Source: CAD feature listing. Evaluate the final solid. Frame: model axes, mm. Face numbers are marked on the shaded views. Coordinates: 2 decimals unless noted, no trailing zeros. Write each loop counter-clockwise with the first axis right and the second up, starting at its lowest first coordinate (ties: lowest second). Pieces come first, ordered by that corner, then holes. Notation, with made-up numbers: (40, 73) - (73, 73) arc R27 cw to (73, 100) - close; hole circle Ø7 at (-17.75, -0.5). An arc over 180 degrees is marked (long way). One line per item, written item: value.
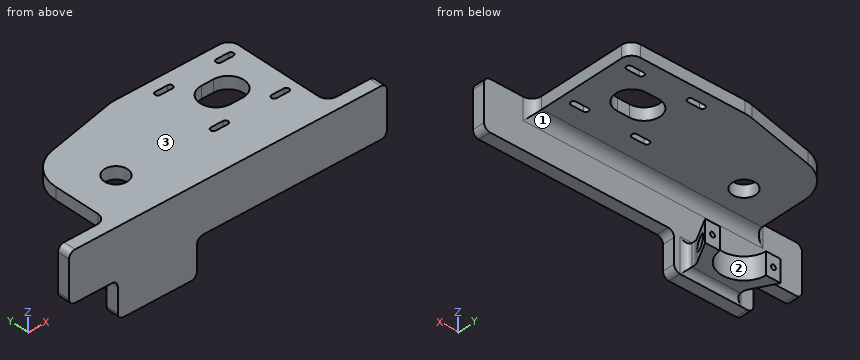
from build123d import *

# Parameters (mm, degrees)
SKETCH1_R           = 9.525
BOSS_EXTRUDE1_DEPTH = 10
SKETCH2_W           = 181
SKETCH2_H           = 100
BOSS_EXTRUDE2_DEPTH = 10
BOSS_EXTRUDE3_DEPTH = 18
SKETCH4_R           = 2
CUT_EXTRUDE1_DEPTH  = 30
SKETCH5_R           = 4
CUT_EXTRUDE2_DEPTH  = 20
CUT_EXTRUDE4_START  = -18
SKETCH8_W           = 62
SKETCH8_H           = 1
CUT_EXTRUDE4_DEPTH  = 18
CUT_EXTRUDE3_REACH  = 171.994
FILLET1_R           = 5
SKETCH9_W           = 40
SKETCH9_H           = 40
BOSS_EXTRUDE5_DEPTH = 10
CUT_EXTRUDE6_DEPTH  = 225.56428954
FILLET2_R           = 5
FILLET3_R           = 5
FILLET4_R           = 8
FILLET5_R           = 30


with BuildPart() as part:
    # Sketch1 → Boss-Extrude1 (new body)
    with BuildSketch(Plane.XY):
        Polygon((146, 57.938160866), (146, -30), (-35, -30), (-35, 40), (49, 57.938160866), align=None)
        Circle(SKETCH1_R, mode=Mode.SUBTRACT)
        with BuildLine():
            Line((101, 33.688160866), (111, 33.688160866))
            ThreePointArc((111, 33.688160866), (124, 20.688160866), (111, 7.688160866))
            Line((111, 7.688160866), (101, 7.688160866))
            ThreePointArc((101, 7.688160866), (88, 20.688160866), (101, 33.688160866))
        make_face(mode=Mode.SUBTRACT)
        with BuildLine():
            Line((86, 43.438160866), (76, 43.438160866))
            ThreePointArc((76, 43.438160866), (73.75, 45.688160866), (76, 47.938160866))
            Line((76, 47.938160866), (86, 47.938160866))
            ThreePointArc((86, 47.938160866), (88.25, 45.688160866), (86, 43.438160866))
        make_face(mode=Mode.SUBTRACT)
        with BuildLine():
            Line((86, -6.561839134), (76, -6.561839134))
            ThreePointArc((76, -6.561839134), (73.75, -4.311839134), (76, -2.061839134))
            Line((76, -2.061839134), (86, -2.061839134))
            ThreePointArc((86, -2.061839134), (88.25, -4.311839134), (86, -6.561839134))
        make_face(mode=Mode.SUBTRACT)
        with BuildLine():
            Line((126, -2.061839134), (136, -2.061839134))
            ThreePointArc((136, -2.061839134), (138.25, -4.311839134), (136, -6.561839134))
            Line((136, -6.561839134), (126, -6.561839134))
            ThreePointArc((126, -6.561839134), (123.75, -4.311839134), (126, -2.061839134))
        make_face(mode=Mode.SUBTRACT)
        with BuildLine():
            Line((126, 47.938160866), (136, 47.938160866))
            ThreePointArc((136, 47.938160866), (138.25, 45.688160866), (136, 43.438160866))
            Line((136, 43.438160866), (126, 43.438160866))
            ThreePointArc((126, 43.438160866), (123.75, 45.688160866), (126, 47.938160866))
        make_face(mode=Mode.SUBTRACT)
    extrude(amount=BOSS_EXTRUDE1_DEPTH)

    # Sketch2 → Boss-Extrude2 (add)
    with BuildSketch(Plane.XZ.offset(30)):
        with Locations((55.5, -40)):
            Rectangle(SKETCH2_W, SKETCH2_H)
    extrude(amount=BOSS_EXTRUDE2_DEPTH)

    # Sketch3 → Boss-Extrude3 (add)
    with BuildSketch(Plane.XY.offset(-55)):
        with BuildLine():
            Line((-31, 0), (-31, -40))
            Line((-31, -40), (31, -40))
            Line((31, -40), (31, 0))
            Line((31, 0), (19, 0))
            ThreePointArc((19, 0), (0, -19), (-19, 0))
            Line((-19, 0), (-31, 0))
        make_face()
    extrude(amount=BOSS_EXTRUDE3_DEPTH)

    # Sketch4 → Cut-Extrude1 (cut)
    with BuildSketch(Plane(origin=(0, 0, 0), x_dir=(1, 0, 0), z_dir=(0, 1, 0))):
        with Locations(Location((-25, 46, 0), (0, 0, 180))):
            Circle(SKETCH4_R)
        with Locations(Location((25, 46, 0), (0, 0, 180))):
            Circle(SKETCH4_R)
    extrude(amount=-CUT_EXTRUDE1_DEPTH, mode=Mode.SUBTRACT)

    # Sketch5 → Cut-Extrude2 (cut)
    with BuildSketch(Plane(origin=(0, -6, 0), x_dir=(1, 0, 0), z_dir=(0, 1, 0))):
        with Locations(Location((25, 46, 0), (0, 0, 180))):
            Circle(SKETCH5_R)
        with Locations(Location((-25, 46, 0), (0, 0, 180))):
            Circle(SKETCH5_R)
    extrude(amount=-CUT_EXTRUDE2_DEPTH, mode=Mode.SUBTRACT)

    # Sketch8 → Cut-Extrude4 (cut)
    with BuildSketch(Plane.XY.offset(-37).offset(CUT_EXTRUDE4_START)):
        with Locations((0, -0.5)):
            Rectangle(SKETCH8_W, SKETCH8_H)
    extrude(amount=CUT_EXTRUDE4_DEPTH, mode=Mode.SUBTRACT)

    # Sketch6 → Cut-Extrude3 (cut, up to next)
    with BuildSketch(Plane(origin=(0, 0, -55), x_dir=(-1, 0, 0), z_dir=(0, 0, -1)), mode=Mode.PRIVATE) as cut_extrude3_sk1:
        Polygon((31, -1), (20, -21), (20, -30), (31, -30), align=None)
    cut_extrude3_tool1 = extrude(cut_extrude3_sk1.sketch, amount=-CUT_EXTRUDE3_REACH, mode=Mode.PRIVATE) & part.part
    # Sketch6 → Cut-Extrude3 (cut, up to next)
    with BuildSketch(Plane(origin=(0, 0, -55), x_dir=(-1, 0, 0), z_dir=(0, 0, -1)), mode=Mode.PRIVATE) as cut_extrude3_sk2:
        Polygon((-31, -1), (-20, -21), (-20, -30), (-31, -30), align=None)
    cut_extrude3_tool2 = extrude(cut_extrude3_sk2.sketch, amount=-CUT_EXTRUDE3_REACH, mode=Mode.PRIVATE) & part.part
    add(cut_extrude3_tool1.solids().sort_by_distance((-26.464912, -19.622807, -55))[0], mode=Mode.SUBTRACT)
    add(cut_extrude3_tool2.solids().sort_by_distance((26.464912, -19.622807, -55))[0], mode=Mode.SUBTRACT)

    # Fillet1
    fillet1_edges = [part.edges().sort_by_distance(p)[0] for p in [
        (-20, -21, -46),
        (-20, -30, -46),
        (20, -30, -46),
        (20, -21, -46),
    ]]
    fillet(fillet1_edges, radius=FILLET1_R)

    # Sketch9 → Boss-Extrude5 (add)
    with BuildSketch(Plane.XZ.offset(40)):
        with Locations((-55, -10)):
            Rectangle(SKETCH9_W, SKETCH9_H)
        with Locations((166, -10)):
            Rectangle(SKETCH9_W, SKETCH9_H)
    extrude(amount=-BOSS_EXTRUDE5_DEPTH)

    # Sketch10 → Cut-Extrude6 (cut, through all)
    with BuildSketch(Plane(origin=(0, -30, 0), x_dir=(1, 0, 0), z_dir=(0, 1, 0))):
        Polygon((30, 30), (30, 60), (-35, 60), (-35, 90), (146, 90), (146, 30), align=None)
    extrude(amount=-CUT_EXTRUDE6_DEPTH, mode=Mode.SUBTRACT)

    # Fillet2
    fillet2_edges = [part.edges().sort_by_distance(p)[0] for p in [
        (-35, -35, -30),
        (-75, -35, -30),
        (-75, -35, 10),
        (186, -35, 10),
        (186, -35, -30),
        (-35, -35, -60),
        (30, -35, -30),
        (30, -35, -60),
    ]]
    fillet(fillet2_edges, radius=FILLET2_R)

    # Fillet3
    fillet3_edges = [part.edges().sort_by_distance(p)[0] for p in [
        (0, -30, -55),
        (0, -30, -37),
    ]]
    fillet(fillet3_edges, radius=FILLET3_R - 0.0001)  # a hair under: the kernel refuses the full size

    # Fillet4
    fillet4_edges = [part.edges().sort_by_distance(p)[0] for p in [
        (-35, -30, 5),
        (146, -30, 5),
        (55.5, -30, 0),
        (146, 57.938160866, 5),
    ]]
    fillet(fillet4_edges, radius=FILLET4_R)

    # Fillet5
    fillet5_edges = [part.edges().sort_by_distance(p)[0] for p in [
        (-35, 40, 5),
        (49, 57.938160866, 5),
    ]]
    fillet(fillet5_edges, radius=FILLET5_R)


solid = part.part
1) Material intervals for line 1 (Z direction, x = 25, y = -10); line 2 (Z direction, x = 25, y = -4.3); line 3 (Z direction, x = 87, y = 6.5), sorted ascending.
Values found:
line 1: -55 to -50, -42 to -37, 0 to 10
line 2: -55 to -48, -44 to -37, 0 to 10
line 3: 0 to 10
2) Draft query along Z for the marked faces 1, 2 and 3. Return one class per face: released by +Z, released by -Z, zero draft, split by the parting line, or undercut.
Values found:
face 1: undercut
face 2: zero draft
face 3: released by +Z
3) Section query B-B on x = 105. Output: boundary loops of the cut face in (y, z), then the cut area to 3 significant figures.
Values found:
outline: (-40, -30) - (-30, -30) - (-30, -8) arc R8 cw to (-22, 0) - (7.69, 0) - (7.69, 10) - (-40, 10) - close; (33.69, 0) - (57.94, 0) - (57.94, 10) - (33.69, 10) - close
area: 1,030 mm2
4) Section query C-C on y = 39.5. Output: boundary loops of the cut face in (x, z).
Values found:
outline: (-23.3, 0) - (146, 0) - (146, 10) - (-23.3, 10) - close
5) Section query A-A on y = 5. Output: boundary loops of the cut face in (x, z), then the cut area to 3 significant figures.
Values found:
outline: (-35, 0) - (-8.11, 0) - (-8.11, 10) - (-35, 10) - close; (8.11, 0) - (146, 0) - (146, 10) - (8.11, 10) - close
area: 1,650 mm2
6) Contact query for flat-ended pins moving along their axis: P1, Ø2, axis at x = 6.5, y = -7, coming from the -Z side; P2, Ø6, axis at x = 38, z = -24.5, coming from the +Y side; P3, Ø13, axis at x = -25, z = -46, coming from the +Y side. Output: stop coordinate, or through.
Values found:
P1: z = 0
P2: y = -30
P3: y = -1
